Geometry: final body of the model. Coordinates: model frame, mm. A direction names the side the tool comes from. Round coordinates to 2 decimals unless told otherwise and drop trailing zeros. Loops run counter-clockwise (first coordinate to the right, second up) from the corner with the lowest first, then second, coordinate; pieces in that order, holes last. Notation, with made-up numbers: M 59,-25.5 L 72,-25.5 A22 ccw 72,-12.5 Z; hole C -29.5,48.5 d2. An arc over 180 degrees is marked long. Write each question's results on one line, items separated by ' | '.
Autodesk Inventor part; units mm, degrees
ref_plane "YZ Plane" through (0, 0, 0) normal (1, 0, 0) x (0, 1, 0)
ref_plane "XZ Plane" through (0, 0, 0) normal (0, 1, 0) x (-1, 0, 0)
ref_plane "XY Plane" through (0, 0, 0) normal (0, 0, 1) x (1, 0, 0)
sketch "Esboço2" plane through (0, 0, 0) normal (0, 0, 1) x (1, 0, 0)
  line L0 (0, 0) -> (9.5, 0)
  line L1 (9.5, 0) -> (9.5, 9.8)
  line L2 (9.5, 9.8) -> (0, 9.8)
  line L3 (0, 9.8) -> (0, 0)
  dimension "d0" = 9.5
  dimension "d1" = 9.8
revolve "Revolução1" add sketch "Esboço2" angle 360 about axis through (0, 0, 0) along (1, 0, 0)
sketch "Esboço3" plane through (0, 0, 0) normal (-1, 0, 0) x (0, 0, 1)
  circle A0 centre (0, 0) radius 1.75
  dimension "d3" = 3.5
extrude "Extrusão1" cut sketch "Esboço3" against normal blind 4.85
sketch "Esboço4" plane through (0, 0, 0) normal (-1, 0, 0) x (0, 0, 1)
  circle A0 centre (0, 0) radius 4.5
  dimension "d6" = 9
extrude "Extrusão2" cut sketch "Esboço4" against normal blind 2
sketch "Esboço8" plane through (9.5, 0, 0) normal (1, 0, 0) x (0, 0, -1)
  circle A0 centre (0, 0) radius 2
  circle A1 centre (0, 0) radius 2.4
  line L0 (2, 0) -> (2, 0.05)
  line L1 (2, 0) -> (1.9994, -0.05)
  line L2 (1.9994, -0.05) -> (2, 0.05)
  line L3 (2, 0.05) -> (2.3777, 0.3266)
  line L4 (1.9994, -0.05) -> (2.3779, -0.3252)
  arc A2 (2.3779, -0.3252) -> (2.3777, 0.3266) centre (0, 0) ccw
  line L5 (2.3777, 0.3266) -> (2.3777, 0.3266)
  line L6 (2.3777, 0.3266) -> (2.3777, 0.3266)
  line L7 (2.3777, 0.3266) -> (2.3777, 0.3266)
  line L8 (2.3779, -0.3252) -> (2.3706, -0.3747)
  line L9 (2.3706, -0.3747) -> (2.3779, -0.3252)
  line L10 (2.3777, 0.3266) -> (2.3777, 0.3266)
  line L11 (2.3777, 0.3266) -> (2.3777, 0.3266)
  line L12 (1.8867, 0.6656) -> (2.1604, 1.0453)
  line L13 (1.917, 0.5703) -> (1.8867, 0.6656)
  line L14 (1.917, 0.5703) -> (2.362, 0.4255)
  line L15 (2.3703, 0.3762) -> (2.362, 0.4255)
  arc A3 (2.362, 0.4255) -> (2.1604, 1.0453) centre (0, 0) ccw
  line L16 (1.5886, 1.216) -> (1.7316, 1.6618)
  line L17 (1.6469, 1.1348) -> (1.5886, 1.216)
  line L18 (1.6469, 1.1348) -> (2.1149, 1.1346)
  line L19 (2.1381, 1.0903) -> (2.1149, 1.1346)
  arc A4 (2.1149, 1.1346) -> (1.7316, 1.6618) centre (0, 0) ccw
  line L20 (1.1351, 1.6474) -> (1.1334, 2.1155)
  line L21 (1.2157, 1.5881) -> (1.1351, 1.6474)
  line L22 (1.2157, 1.5881) -> (1.6608, 1.7326)
  line L23 (1.6965, 1.6976) -> (1.6608, 1.7326)
  arc A5 (1.6608, 1.7326) -> (1.1334, 2.1155) centre (0, 0) ccw
  line L24 (0.5705, 1.9176) -> (0.4241, 2.3622)
  line L25 (0.6654, 1.8861) -> (0.5705, 1.9176)
  line L26 (0.6654, 1.8861) -> (1.0441, 2.161)
  line L27 (1.0889, 2.1388) -> (1.0441, 2.161)
  arc A6 (1.0441, 2.161) -> (0.4241, 2.3622) centre (0, 0) ccw
  line L28 (-0.05, 2) -> (-0.3266, 2.3777)
  line L29 (0.05, 1.9994) -> (-0.05, 2)
  line L30 (0.05, 1.9994) -> (0.3252, 2.3779)
  line L31 (0.3747, 2.3706) -> (0.3252, 2.3779)
  arc A7 (0.3252, 2.3779) -> (-0.3266, 2.3777) centre (0, 0) ccw
  line L32 (-0.6656, 1.8867) -> (-1.0453, 2.1604)
  line L33 (-0.5703, 1.917) -> (-0.6656, 1.8867)
  line L34 (-0.5703, 1.917) -> (-0.4255, 2.362)
  line L35 (-0.3762, 2.3703) -> (-0.4255, 2.362)
  arc A8 (-0.4255, 2.362) -> (-1.0453, 2.1604) centre (0, 0) ccw
  line L36 (-1.216, 1.5886) -> (-1.6618, 1.7316)
  line L37 (-1.1348, 1.6469) -> (-1.216, 1.5886)
  line L38 (-1.1348, 1.6469) -> (-1.1346, 2.1149)
  line L39 (-1.0903, 2.1381) -> (-1.1346, 2.1149)
  arc A9 (-1.1346, 2.1149) -> (-1.6618, 1.7316) centre (0, 0) ccw
  line L40 (-1.6474, 1.1351) -> (-2.1155, 1.1334)
  line L41 (-1.5881, 1.2157) -> (-1.6474, 1.1351)
  line L42 (-1.5881, 1.2157) -> (-1.7326, 1.6608)
  line L43 (-1.6976, 1.6965) -> (-1.7326, 1.6608)
  arc A10 (-1.7326, 1.6608) -> (-2.1155, 1.1334) centre (0, 0) ccw
  line L44 (-1.9176, 0.5705) -> (-2.3622, 0.4241)
  line L45 (-1.8861, 0.6654) -> (-1.9176, 0.5705)
  line L46 (-1.8861, 0.6654) -> (-2.161, 1.0441)
  line L47 (-2.1388, 1.0889) -> (-2.161, 1.0441)
  arc A11 (-2.161, 1.0441) -> (-2.3622, 0.4241) centre (0, 0) ccw
  line L48 (-2, -0.05) -> (-2.3777, -0.3266)
  line L49 (-1.9994, 0.05) -> (-2, -0.05)
  line L50 (-1.9994, 0.05) -> (-2.3779, 0.3252)
  line L51 (-2.3706, 0.3747) -> (-2.3779, 0.3252)
  arc A12 (-2.3779, 0.3252) -> (-2.3777, -0.3266) centre (0, 0) ccw
  line L52 (-1.8867, -0.6656) -> (-2.1604, -1.0453)
  line L53 (-1.917, -0.5703) -> (-1.8867, -0.6656)
  line L54 (-1.917, -0.5703) -> (-2.362, -0.4255)
  line L55 (-2.3703, -0.3762) -> (-2.362, -0.4255)
  arc A13 (-2.362, -0.4255) -> (-2.1604, -1.0453) centre (0, 0) ccw
  line L56 (-1.5886, -1.216) -> (-1.7316, -1.6618)
  line L57 (-1.6469, -1.1348) -> (-1.5886, -1.216)
  line L58 (-1.6469, -1.1348) -> (-2.1149, -1.1346)
  line L59 (-2.1381, -1.0903) -> (-2.1149, -1.1346)
  arc A14 (-2.1149, -1.1346) -> (-1.7316, -1.6618) centre (0, 0) ccw
  line L60 (-1.1351, -1.6474) -> (-1.1334, -2.1155)
  line L61 (-1.2157, -1.5881) -> (-1.1351, -1.6474)
  line L62 (-1.2157, -1.5881) -> (-1.6608, -1.7326)
  line L63 (-1.6965, -1.6976) -> (-1.6608, -1.7326)
  arc A15 (-1.6608, -1.7326) -> (-1.1334, -2.1155) centre (0, 0) ccw
  line L64 (-0.5705, -1.9176) -> (-0.4241, -2.3622)
  line L65 (-0.6654, -1.8861) -> (-0.5705, -1.9176)
  line L66 (-0.6654, -1.8861) -> (-1.0441, -2.161)
  line L67 (-1.0889, -2.1388) -> (-1.0441, -2.161)
  arc A16 (-1.0441, -2.161) -> (-0.4241, -2.3622) centre (0, 0) ccw
  line L68 (0.05, -2) -> (0.3266, -2.3777)
  line L69 (-0.05, -1.9994) -> (0.05, -2)
  line L70 (-0.05, -1.9994) -> (-0.3252, -2.3779)
  line L71 (-0.3747, -2.3706) -> (-0.3252, -2.3779)
  arc A17 (-0.3252, -2.3779) -> (0.3266, -2.3777) centre (0, 0) ccw
  line L72 (0.6656, -1.8867) -> (1.0453, -2.1604)
  line L73 (0.5703, -1.917) -> (0.6656, -1.8867)
  line L74 (0.5703, -1.917) -> (0.4255, -2.362)
  line L75 (0.3762, -2.3703) -> (0.4255, -2.362)
  arc A18 (0.4255, -2.362) -> (1.0453, -2.1604) centre (0, 0) ccw
  line L76 (1.216, -1.5886) -> (1.6618, -1.7316)
  line L77 (1.1348, -1.6469) -> (1.216, -1.5886)
  line L78 (1.1348, -1.6469) -> (1.1346, -2.1149)
  line L79 (1.0903, -2.1381) -> (1.1346, -2.1149)
  arc A19 (1.1346, -2.1149) -> (1.6618, -1.7316) centre (0, 0) ccw
  line L80 (1.6474, -1.1351) -> (2.1155, -1.1334)
  line L81 (1.5881, -1.2157) -> (1.6474, -1.1351)
  line L82 (1.5881, -1.2157) -> (1.7326, -1.6608)
  line L83 (1.6976, -1.6965) -> (1.7326, -1.6608)
  arc A20 (1.7326, -1.6608) -> (2.1155, -1.1334) centre (0, 0) ccw
  line L84 (1.9176, -0.5705) -> (2.3622, -0.4241)
  line L85 (1.8861, -0.6654) -> (1.9176, -0.5705)
  line L86 (1.8861, -0.6654) -> (2.161, -1.0441)
  line L87 (2.1388, -1.0889) -> (2.161, -1.0441)
  arc A21 (2.161, -1.0441) -> (2.3622, -0.4241) centre (0, 0) ccw
  point P0 (1.9998, 0.025)
  point P1 (1.8942, 0.6418)
  point P2 (1.6032, 1.1957)
  point P3 (1.1553, 1.6326)
  point P4 (0.5942, 1.9097)
  point P5 (-0.025, 1.9998)
  point P6 (-0.6418, 1.8942)
  point P7 (-1.1957, 1.6032)
  point P8 (-1.6326, 1.1553)
  point P9 (-1.9097, 0.5942)
  point P10 (-1.9998, -0.025)
  point P11 (-1.8942, -0.6418)
  point P12 (-1.6032, -1.1957)
  point P13 (-1.1553, -1.6326)
  point P14 (-0.5942, -1.9097)
  point P15 (0.025, -1.9998)
  point P16 (0.6418, -1.8942)
  point P17 (1.1957, -1.6032)
  point P18 (1.6326, -1.1553)
  point P19 (1.9097, -0.5942)
  dimension "d35" = 4
  dimension "d36" = 4.8
  dimension "d37" = 0.05
  dimension "d38" = 0.05
  dimension "d39" = 0.05
  dimension "d44" = 360
extrude "Extrusão3" cut sketch "Esboço8" against normal blind 3.5 contours A0 | A0 L14 A1 L3 | L4 A1 L84 A0 | A0 L18 A1 L12 | L86 A1 L80 A0 | A0 L22 A1 L16 | L82 A1 L76 A0 | A0 L26 A1 L20 | L78 A1 L72 A0 | A0 L30 A1 L24 | L74 A1 L68 A0 | A0 L34 A1 L28 | L70 A1 L64 A0 | A0 L38 A1 L32 | L66 A1 L60 A0 | A0 L42 A1 L36 | L62 A1 L56 A0 | A0 L46 A1 L40 | L58 A1 L52 A0 | A0 L50 A1 L44 | L54 A1 L48 A0
sketch "Esboço9" plane through (9.5, 0, 0) normal (1, 0, 0) x (0, 0, -1)
  point P0 (0, 0)
properties part number "roda certa"
1. Section D-D (z = 3.5). Output: boundary loops of the cut face in (x, y).
Answer key:
outline: M 0,-9.15 L 9.5,-9.15 L 9.5,9.15 L 0,9.15 L 0,2.83 L 2,2.83 L 2,-2.83 L 0,-2.83 Z
2. Pin query (flat end, axial travel): P1, Ø0.5, axis at x = 8, y = -2, coming from the +Z side; P2, Ø3, axis at y = 0, z = 0, coming from the -X side; P3, Ø2, axis at x = 4, z = 2.5, coming from the +Y side. Return the tip coordinate at first contact, or that it passes through.
Answer key:
P1: stops at z = 9.64 | P2: stops at x = 4.85 | P3: stops at y = 9.68
3. Access query for faces 1 (the face through (2, -2, 0)), 2 (the face through (6, 0, 0)), 3 (the face through (0, 4.2, -2)). Directions: +Z, -Z, +X, -X, +Y, -Y. A direction counts if a zero-diameter tool reaches every point of the face in a straight line with its end or side. Return the directions, or none.
Answer key:
face 1: -X | face 2: +X | face 3: +Z, -Z, -X, +Y, -Y
4. Section A-A (x = 3.5). Output: boundary loops of the cut face in (y, z), then the cut area to 3 significant figures.
Answer key:
outline: C 0,0 d19.6; hole C 0,0 d3.5 | area: 292 mm²
5. Draft query along Y for faces 4 (the face through (9.5, 2, -2)), 5 (the face through (4.684, -2.124, 9.567)), 6 (the face through (0.99, 4.46, -0.59)). Return one class per face: pulls with the +Y half, pulls with the -Y half, needs draft (parallel to the pull), parting line crosses it, or undercut.
Answer key:
face 4: needs draft | face 5: parting line crosses it | face 6: undercut
6. Section B-B (z = -3.25). Output: boundary loops of the cut face in (x, y), then the cut area to 3 significant figures.
Answer key:
outline: M 0,-9.25 L 9.5,-9.25 L 9.5,9.25 L 0,9.25 L 0,3.11 L 2,3.11 L 2,-3.11 L 0,-3.11 Z | area: 163 mm²
7. Section C-C (y = -5). Output: boundary loops of the cut face in (x, z), then the cut area to 3 significant figures.
Answer key:
outline: M 0,-8.43 L 9.5,-8.43 L 9.5,8.43 L 0,8.43 Z | area: 160 mm²
8. Ray query, probe 1 along Y at (x, z) = (3.75, 0.25); probe 2 along Y at (x, z) = (9, -2.25); probe 3 along Y at (x, z) = (3, 1). Return the intervals inside material, ascending.
Answer key:
probe 1: y = -9.8 to -1.73, 1.73 to 9.8 | probe 2: y = -9.54 to -0.46, -0.23 to 0.23, 0.46 to 9.54 | probe 3: y = -9.75 to -1.44, 1.44 to 9.75
